Part print with two shaded views. Sizes in mm from the minimum x, y, z corner. Give positions to 0.01 mm unless a question says otherwise; leave off trailing zeros. Write each loop counter-clockwise with the first axis right and the second up, starting at its lowest first coordinate (ties: lowest second). Pieces come first, ordered by that corner, then holes. Notation, with made-up numbers: (50, 79) - (84, 79) arc R14 ccw to (84, 105) - close; hole circle Ø7 at (-6, 42). An arc over 180 degrees is marked (long way). One line per item, written item: value. Start each with the question number.
(1) Cut at A-A, the plane y = 4.95. List the corners of the cut face in (x, z).
(2) Cut at B-B, the plane x = 62. List the corners of the cut face in (y, z), and give its area (3 significant figures).
(3) Cut at C-C, the plane z = 80. List the corners of the cut face in (x, y), and give its area (3 significant figures).
(4) Cut at D-D, the plane z = 26. List the corners of the cut face in (x, y).
(5) Drop a flat-ended pin along its axis: P1, Ø3.5, axis at x = 10, z = 10, coming from the +Y side. Give the stop position or say it passes through.
(6) Probe L1, parallel to Z at x = 62, y = 0.85; L2, parallel to X at y = 1.7, z = 10; L3, parallel to Z at x = 10, y = 5.05. List the from-to ranges inside material, lowest first.
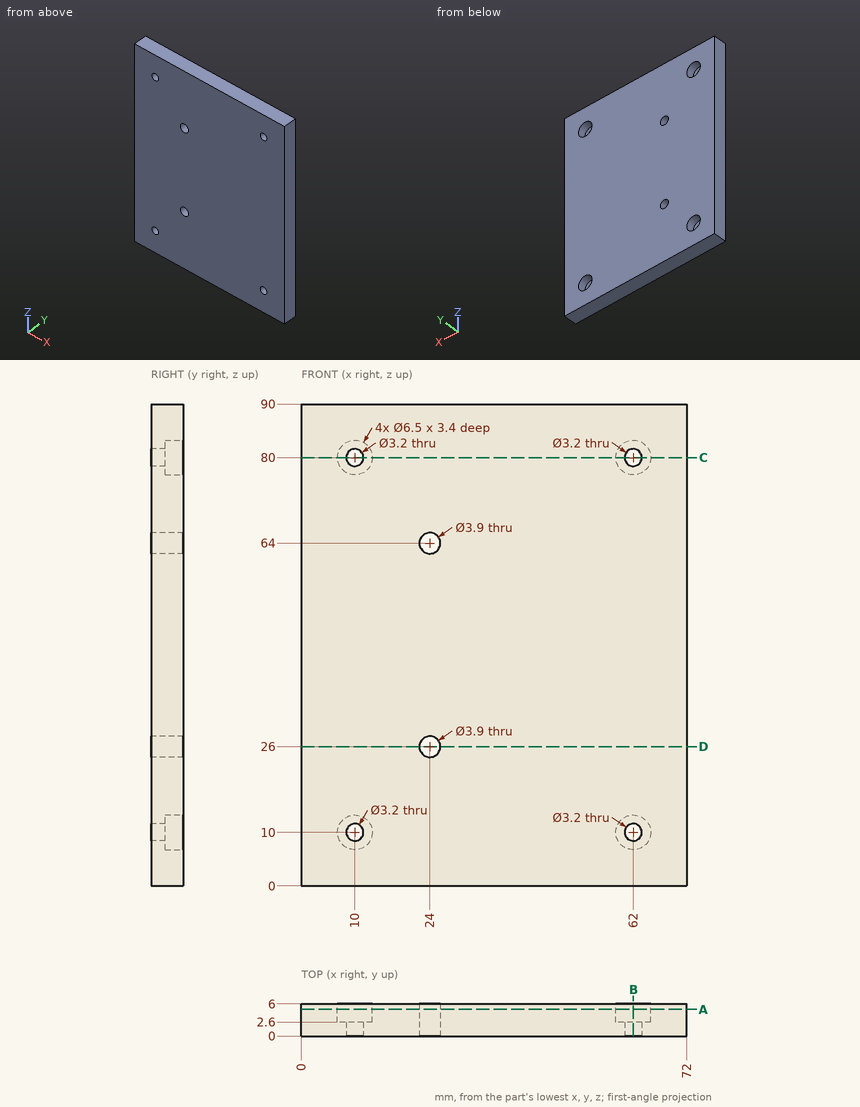
Answers follow:
1. outline: (0, 0) - (72, 0) - (72, 90) - (0, 90) - close; hole circle Ø6.5 at (10, 10); hole circle Ø6.5 at (10, 80); hole circle Ø3.9 at (24, 26); hole circle Ø3.9 at (24, 64); hole circle Ø6.5 at (62, 10); hole circle Ø6.5 at (62, 80)
2. outline: (0, 0) - (6, 0) - (6, 6.75) - (2.6, 6.75) - (2.6, 8.4) - (0, 8.4) - close; (0, 11.6) - (2.6, 11.6) - (2.6, 13.25) - (6, 13.25) - (6, 76.75) - (2.6, 76.75) - (2.6, 78.4) - (0, 78.4) - close; (0, 81.6) - (2.6, 81.6) - (2.6, 83.25) - (6, 83.25) - (6, 90) - (0, 90) - close
2. area: 479 mm²
3. outline: (0, 0) - (8.4, 0) - (8.4, 2.6) - (6.75, 2.6) - (6.75, 6) - (0, 6) - close; (11.6, 0) - (60.4, 0) - (60.4, 2.6) - (58.75, 2.6) - (58.75, 6) - (13.25, 6) - (13.25, 2.6) - (11.6, 2.6) - close; (63.6, 0) - (72, 0) - (72, 6) - (65.25, 6) - (65.25, 2.6) - (63.6, 2.6) - close
3. area: 371 mm²
4. outline: (0, 0) - (22.05, 0) - (22.05, 6) - (0, 6) - close; (25.95, 0) - (72, 0) - (72, 6) - (25.95, 6) - close
5. P1: stops at y = 2.6
6. L1: z = 0 to 8.4, 11.6 to 78.4, 81.6 to 90
6. L2: x = 0 to 8.4, 11.6 to 60.4, 63.6 to 72
6. L3: z = 0 to 6.75, 13.25 to 76.75, 83.25 to 90
